Check sheet for the modelled part. Datum: model origin and axes. Units: mm. Face numbers are marked on the shaded views. A direction names the side the tool comes from. Give positions to 0.01 mm unless a question says otherwise; leave off trailing zeros. Order: outer loops, then holes, each group sorted by start corner. A loop starts at its lowest first (then second) coordinate and runs counter-clockwise, first axis right, second up.
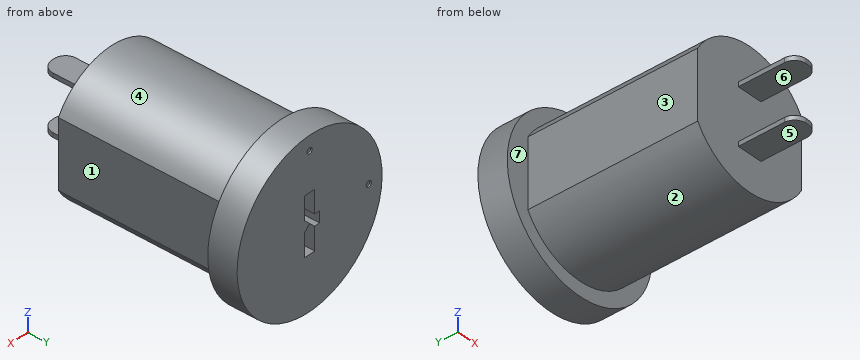
```python
from build123d import *

# Parameters (mm, degrees)
SKETCH2_W           = 3.302901435
SKETCH2_H           = 13.888103622
CUT_EXTRUDE1_DEPTH  = 15.0276
SKETCH3_W           = 2.2606
SKETCH3_H           = 0.3937
BOSS_EXTRUDE1_DEPTH = 5.08
FILLET1_R           = 1.016
CUT_EXTRUDE2_DEPTH  = 2.54
SKETCH5_R           = 0.254
CUT_EXTRUDE3_DEPTH  = 0.127


with BuildPart() as part:
    # Sketch1 → Revolve1 (revolve)
    with BuildSketch(Plane.XY, mode=Mode.PRIVATE) as revolve1_sk:
        Polygon((0, 17.6276), (-7.25, 17.6276), (-7.25, 15.0276), (-6, 15.0276), (-6, 0), (0, 0), align=None)
    revolve(revolve1_sk.sketch.rotate(Axis((0, 19.222907737, 0), (0, -1, 0)), 270), axis=Axis((0, 19.222907737, 0), (0, -1, 0)))

    # Sketch2 → Cut-Extrude1 (cut)
    with BuildSketch(Plane.XZ):
        with Locations((-6.851450718, -0.431101593)):
            Rectangle(SKETCH2_W, SKETCH2_H)
        with Locations((6.851450718, -0.431101593)):
            Rectangle(SKETCH2_W, SKETCH2_H)
    extrude(amount=-CUT_EXTRUDE1_DEPTH, mode=Mode.SUBTRACT)

    # Sketch3 → Boss-Extrude1 (add)
    with BuildSketch(Plane.XZ):
        with Locations((0, 2.25315)):
            Rectangle(SKETCH3_W, SKETCH3_H)
        with Locations((0, -2.64685)):
            Rectangle(SKETCH3_W, SKETCH3_H)
    extrude(amount=BOSS_EXTRUDE1_DEPTH)

    # Fillet1
    fillet1_edges = [part.edges().sort_by_distance(p)[0] for p in [
        (1.1303, -5.08, 2.25315),
        (-1.1303, -5.08, 2.25315),
        (1.1303, -5.08, -2.64685),
        (-1.1303, -5.08, -2.64685),
    ]]
    fillet(fillet1_edges, radius=FILLET1_R)

    # Sketch4 → Cut-Extrude2 (cut)
    with BuildSketch(Plane(origin=(0, 17.6276, 0), x_dir=(1, 0, 0), z_dir=(0, 1, 0))):
        Polygon((0.508, 2.54), (0.508, 0.506703339), (0, 0), (0.508, -0.509299979), (0.508, -2.54), (-0.508, -2.54), (-0.508, -0.508), (-1.003091962, -0.508), (-1.003091962, 0.508), (-0.508, 0.508), (-0.508, 2.54), align=None)
    extrude(amount=-CUT_EXTRUDE2_DEPTH, mode=Mode.SUBTRACT)

    # Sketch5 → Cut-Extrude3 (cut)
    with BuildSketch(Plane(origin=(0, 17.6276, 0), x_dir=(1, 0, 0), z_dir=(0, 1, 0))):
        with Locations(Location((-5.91604032, 0, 0), (0, 0, 270))):
            Circle(SKETCH5_R)
        with Locations(Location((0, -5.969098978, 0), (0, 0, 270))):
            Circle(SKETCH5_R)
    extrude(amount=-CUT_EXTRUDE3_DEPTH, mode=Mode.SUBTRACT)


solid = part.part
```
(1) Cross-section at B-B on z = -5. Enter the section's corners in (x, y), then the cut area to 3 significant figures.
Response values:
outline: (-5.25, 15.03) - (-3.32, 15.03) - (-3.32, 0) - (3.32, 0) - (3.32, 15.03) - (5.25, 15.03) - (5.25, 17.63) - (-5.25, 17.63) - close
area: 127 mm2
(2) Release check for a two-part mould opening along Z. For the marked faces 4, 5, 6 and 7 record: released by +Z, released by -Z, zero draft, split by the parting line, or undercut.
Response values:
face 4: released by +Z
face 5: released by -Z
face 6: undercut
face 7: zero draft
(3) Set-up check for the marked faces 1, 2 and 3: record each of +Z, -Z, +X, -X, +Y, -Y from which the full face is reachable in a straight line by a thin tool's end or side.
Response values:
face 1: +Z, -Z, +X, -Y
face 2: -Z, -Y
face 3: +Z, -Z, -X, -Y
(4) Material ranges on L1, parallel to Z at x = -0.5, y = -2; L2, parallel to Y at x = -5, z = -1.5; L3, parallel to X at y = 1, z = 0.75, recorded low to high.
Response values:
L1: z = -2.84 to -2.45, 2.06 to 2.45
L2: y = 0 to 17.63
L3: x = -5.2 to 5.2
(5) Cross-section at C-C on x = 3. Enter the section's corners in (y, z).
Response values:
outline: (0, -5.2) - (15.03, -5.2) - (15.03, -6.6) - (17.63, -6.6) - (17.63, 6.6) - (15.03, 6.6) - (15.03, 5.2) - (0, 5.2) - close
(6) Cross-section at A-A on y = -2.25. Enter the section's corners in (x, z), then the cut area to 3 significant figures.
Response values:
outline: (-1.13, -2.84) - (1.13, -2.84) - (1.13, -2.45) - (-1.13, -2.45) - close; (-1.13, 2.06) - (1.13, 2.06) - (1.13, 2.45) - (-1.13, 2.45) - close
area: 1.78 mm2
(7) Gauge pin test, flat ends, axial feed: pin 1 Ø5 at (y, z) = (-1.5, 0.5) entering from +X; pin 2 Ø3 at (x, y) = (1.5, 8.5) entering from -Z; pin 3 Ø0.5 at (x, y) = (-1, 17) entering from -Z. Record the tip position at first contact, or that the pin passes through.
Response values:
pin 1: stops at x = 5.2
pin 2: stops at z = -6
pin 3: stops at z = -7.21
(8) Cross-section at D-D on y = 0.5. Enter the section's corners in (x, z).
Response values:
outline: (-5.2, -2.99) arc R6 ccw to (5.2, -2.99) - (5.2, 2.99) arc R6 ccw to (-5.2, 2.99) - close
